Work out the finished part from the listing and answer in its coordinate system (mm). A direction names the side the tool comes from. Round coordinates to 2 decimals unless told otherwise and drop trailing zeros. Return JSON: item names as keys, results as strings.
from build123d import *

# Parameters (mm, degrees)
F1_DEPTH = 40.2336
F0_R     = 10.16
F2_DEPTH = 15.7734
F3_R     = 3.302


with BuildPart() as f1:
    # F0 (on Front) → F1 (new body)
    with BuildSketch(Plane.XZ):
        with BuildLine():
            ThreePointArc((-47.222857, -28.021934), (-30.722388, -18.119866), (-24.242661, 0))
            ThreePointArc((-24.242661, 0), (-30.901637, 18.336262), (-47.775014, 28.126541))
            ThreePointArc((-47.775014, 28.126541), (-81.39128, -0.28099), (-47.222857, -28.021934))
        make_face()
        with BuildLine():
            ThreePointArc((-39.369896, -4.826), (-67.105161, 0), (-39.369896, 4.826))
            Line((-39.369896, 4.826), (-34.288361, 4.826))
            Line((-34.288361, 4.826), (-34.288361, 0))
            Line((-34.288361, 0), (-34.288361, -4.826))
            Line((-34.288361, -4.826), (-39.369896, -4.826))
        make_face(mode=Mode.SUBTRACT)
    extrude(amount=F1_DEPTH)

    # F0 (on Front) → F2 (join)
    with BuildSketch(Plane.XZ):
        with BuildLine():
            ThreePointArc((-47.775014, 28.126541), (-30.901637, 18.336262), (-24.242661, 0))
            ThreePointArc((-24.242661, 0), (-30.722388, -18.119866), (-47.222857, -28.021934))
            Line((-47.222857, -28.021934), (4.517132, -18.751381))
            ThreePointArc((4.517132, -18.751381), (-17.892661, 0.001001), (4.519103, 18.751028))
            Line((4.519103, 18.751028), (-47.775014, 28.126541))
        make_face()
        with BuildLine():
            ThreePointArc((20.207339, 0), (15.768022, 12.224174), (4.519103, 18.751028))
            ThreePointArc((4.519103, 18.751028), (-17.892661, 0.001001), (4.517132, -18.751381))
            ThreePointArc((4.517132, -18.751381), (15.767379, -12.224942), (20.207339, 0))
        make_face()
        with Locations((1.157339, 0)):
            Circle(F0_R, mode=Mode.SUBTRACT)
    extrude(amount=F2_DEPTH)

    # F3
    f3_edges = [f1.edges().sort_by_distance(p)[0] for p in [
        (-58.412466, -40.2336, 28.021934),
    ]]
    fillet(f3_edges, radius=F3_R)


solid = f1.part
Item 1: The mould has two halves that part along X. Classify faces 1 (the flat face through (-21.262, -7.776, 23.373)), 2 (the cylindrical face through (10.85, -7.78, 3.05)), 3 (the flat face through (-42, -40.234, -11)): pulls with the +X half, pulls with the -X half, needs draft (parallel to the pull), parting line crosses it, or undercut.
Output:
{"face 1": "pulls with the +X half", "face 2": "undercut", "face 3": "needs draft"}
Item 2: Which of the six approach directions +Z, -Z, +X, -X, +Y, -Y give full straight-line access (tool end or side, diameter ignored) to faces 4 (the flat face through (-34.288, -20, 0)), 5 (the flat face through (-31, 0, 0))?
Output:
{"face 4": "+Y, -Y", "face 5": "+Z, -Z, +X, -X, +Y"}
Item 3: Find section A-A (y = -10). State how many separate pieces and enclosed holes the cut face has, plus the area to 3 significant figures.
Output:
{"separate pieces": "1", "enclosed holes": "2", "area": "3,450 mm^2"}
Item 4: Each of these flat-tipped pins is pushed along its axis until it touches: pin 1 (8 mm diameter, centred on y = -11.5, z = -21, fed in from +X); pin 2 (5 mm diameter, centred on x = -27.5, y = -14, fed in from +Z); pin 3 (5 mm diameter, centred on y = -20, z = -8.5, fed in from +X); pin 4 (17 mm diameter, centred on x = -52.82, z = 0, fed in from -Y). Where does it stop, or does it pass through?
Output:
{"pin 1": "stops at x = 9.75", "pin 2": "stops at z = 24.94", "pin 3": "stops at x = -24.88", "pin 4": "passes through"}
Item 5: Consider line 1 along X through (y, z) = (-27, 0); line 2 along X through (y, z) = (-9, 9); line 3 along Z through (x, y) = (-55.5, -2). Determine where each line is inside the solid, lowest interval first. Write a range as [from, to].
Output:
{"line 1": "x = [-81.39, -67.11], [-34.29, -24.24]", "line 2": "x = [-79.94, -63.91], [-41.72, -3.56], [5.87, 17.95]", "line 3": "z = [-28.45, -14.03], [14.03, 28.45]"}
